The model under review builds one solid part; all positions refer to its coordinate system, in mm. Give positions to 0.01 mm unless a question says otherwise; leave off trailing zeros. Loops run counter-clockwise (first coordinate to the right, second up) from the corner with the lowest first, then second, coordinate; pieces in that order, holes last. Notation, with made-up numbers: M -5,84.25 L 31,84.25 A15 ccw 31,95.25 Z; hole C 88,-25 d7. An arc over 180 degrees is marked long. Write item = value, one per line. Start each with the question number.
1. We need section A-A on y = 0. Give the boundary of the cut face in (x, z) (3 decimals), then the cut area to 3 significant figures.
2. We need section D-D on z = 59.5. Give the boundary of the cut face in (x, y) (3 decimals).
3. We need section C-C on z = 145. Give the boundary of the cut face in (x, y) (3 decimals), then the cut area to 3 significant figures.
4. Draft analysis for pull direction Z (two halves, no side actions). For faces 1 (the face through (0.751, -10.21, 147.385)), 2 (the face through (0, 9, 0)), 3 (the face through (-7.003, -5.37, 78.88)), state which applies: pulls with the +Z half, pulls with the -Z half, needs draft (parallel to the pull), parting line crosses it, or undercut.
5. We need section B-B on x = 0. Give the boundary of the cut face in (y, z) (3 decimals).
6. Wall thickness on line 1 along Z through (x, y) = (0, 9.35); line 2 along Y through (x, z) = (0.5, 133); line 3 along Z through (x, y) = (1.75, 10.75): over which ranges is each line inside the solid? List them lowest first. Write a range as from..to.
7. For pin 1 (1 mm diameter, centred on x = 9, z = 79.5, fed in from -Y); pin 2 (1.5 mm diameter, centred on y = 3, z = 132, fed in from +X); pin 3 (2 mm diameter, centred on y = 3.5, z = 53, fed in from +X), all flat-tipped, find the tip position at first contact; note any pin that passes through.
from build123d import *

# Parameters (mm, degrees)
SKETCH1_R               = 12
BOSS_EXTRUDE1_DEPTH     = 160
SHELL1_T                = -3.175
SKETCH2_R               = 2.5
CUT_EXTRUDE1_DEPTH      = 161.897482889
CUT_EXTRUDE1_DEPTH_BACK = 161.897482889


with BuildPart() as part:
    # Sketch1 → Boss-Extrude1 (new body)
    with BuildSketch(Plane.XY):
        Circle(SKETCH1_R)
    extrude(amount=BOSS_EXTRUDE1_DEPTH)

    # Shell1
    shell1_openings = [part.faces().sort_by_distance(p)[0] for p in [
        (0, 0, 160),
        (0, 0, 0),
    ]]
    offset(amount=SHELL1_T, openings=shell1_openings, kind=Kind.INTERSECTION)

    # Sketch2 → Cut-Extrude1 (cut, two sides)
    with BuildSketch(Plane(origin=(0, 0, 0), x_dir=(1, 0, 0), z_dir=(0, 1, 0))) as cut_extrude1_sk:
        with Locations(Location((0, -15, 0), (0, 0, 270))):
            Circle(SKETCH2_R)
        with Locations(Location((0, -145, 0), (0, 0, 270))):
            Circle(SKETCH2_R)
    extrude(amount=CUT_EXTRUDE1_DEPTH, mode=Mode.SUBTRACT)
    extrude(cut_extrude1_sk.sketch, amount=-CUT_EXTRUDE1_DEPTH_BACK, mode=Mode.SUBTRACT)


solid = part.part
Final values:
q1.outline = M -12,0 L -8.825,0 L -8.825,160 L -12,160 Z; M 8.825,0 L 12,0 L 12,160 L 8.825,160 Z
q1.area = 1,020 mm²
q2.outline = C 0,0 d24; hole C 0,0 d17.65
q3.outline = M -2.5,-11.737 L -2.5,-8.463 A8.825 cw -2.5,8.463 L -2.5,11.737 A12 ccw Z; M 2.5,-11.737 A12 ccw 2.5,11.737 L 2.5,8.463 A8.825 cw 2.5,-8.463 Z
q3.area = 176 mm²
q4.face_1 = undercut
q4.face_2 = pulls with the -Z half
q4.face_3 = needs draft
q5.outline = M -12,0 L -8.825,0 L -8.825,12.5 L -12,12.5 Z; M -12,17.5 L -8.825,17.5 L -8.825,142.5 L -12,142.5 Z; M -12,147.5 L -8.825,147.5 L -8.825,160 L -12,160 Z; M 8.825,0 L 12,0 L 12,12.5 L 8.825,12.5 Z; M 8.825,17.5 L 12,17.5 L 12,142.5 L 8.825,142.5 Z; M 8.825,147.5 L 12,147.5 L 12,160 L 8.825,160 Z
q6.line_1 = 0..12.5, 17.5..142.5, 147.5..160
q6.line_2 = -11.99..-8.81, 8.81..11.99
q6.line_3 = 0..13.21, 16.79..143.21, 146.79..160
q7.pin_1 = -8.47
q7.pin_2 = 11.79
q7.pin_3 = 11.74
